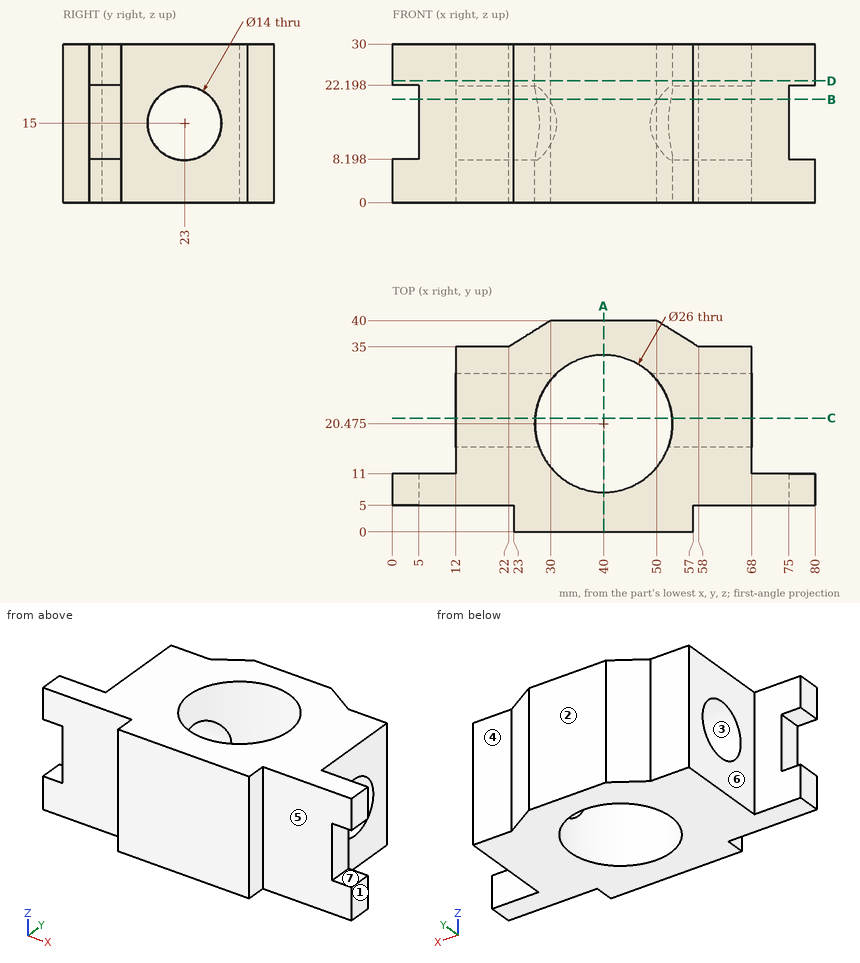
Check sheet for the drawn part. Datum: minimum x, y, z corner. Units: mm. A direction names the side the tool comes from. Coordinates: 2 decimals unless noted, no trailing zeros. Loops run counter-clockwise (first coordinate to the right, second up) from the corner with the lowest first, then second, coordinate; pieces in that order, holes last. Notation, with made-up numbers: (-26.5, 81.25) -> (-20.5, 81.25) arc R16 cw to (-20.5, 103.25) -> close; hole circle Ø7 at (44, -38.75). An arc over 180 degrees is marked (long way). Write each question's results on one line, items separated by ' | '.
Item 1: Mould release check, pull along Y, two halves, no side actions. Record for the marked faces 1, 2 and 3: +Y half, -Y half, draft (parallel to the pull), parting line (faces both ways), or undercut.
Found:
face 1: draft | face 2: +Y half | face 3: undercut
Item 2: Tool access check on the marked faces 4, 5, 6 and 7. Record the directions out of +Z, -Z, +X, -X, +Y, -Y that give a thin tool (end or side, any length) a straight path to the whole face; none if there is none.
Found:
face 4: +Z, -Z, +X, +Y | face 5: +Z, -Z, +X, -Y | face 6: +Z, -Z, -X, +Y | face 7: +X, +Y, -Y
Item 3: Section check C-C, the plane y = 21.5. Enter the section's corners in (x, z).
Found:
outline: (12, 0) -> (27.04, 0) -> (27.04, 8.16) -> (12, 8.16) -> close; (12, 21.84) -> (27.04, 21.84) -> (27.04, 30) -> (12, 30) -> close; (52.96, 0) -> (68, 0) -> (68, 8.16) -> (52.96, 8.16) -> close; (52.96, 21.84) -> (68, 21.84) -> (68, 30) -> (52.96, 30) -> close
Item 4: Material ranges on L1, parallel to Y at x = 40, z = 16 (1 decimal); L2, parallel to Z at x = 21, y = 23; L3, parallel to Y at x = 19.5, z = 25, recorded low to high.
Found:
L1: y = 0 to 7.5, 33.5 to 40 | L2: z = 0 to 8, 22 to 30 | L3: y = 5 to 35
Item 5: Section check A-A, the plane x = 40. Enter the section's corners in (y, z) (1 decimal).
Found:
outline: (0, 0) -> (7.5, 0) -> (7.5, 30) -> (0, 30) -> close; (33.5, 0) -> (40, 0) -> (40, 30) -> (33.5, 30) -> close
Item 6: Section check D-D, the plane z = 23. Enter the section's corners in (x, y) (1 decimal), plus the area to 3 significant figures.
Found:
outline: (0, 5) -> (23, 5) -> (23, 0) -> (57, 0) -> (57, 5) -> (80, 5) -> (80, 11) -> (68, 11) -> (68, 35) -> (58, 35) -> (50, 40) -> (30, 40) -> (22, 35) -> (12, 35) -> (12, 11) -> (0, 11) -> close; hole circle Ø26 at (40, 20.5) | area: 1,600 mm2
Item 7: Gauge pin test, flat ends, axial feed: pin 1 (10 mm diameter, centred on y = 25, z = 9.5, fed in from -X); pin 2 (5 mm diameter, centred on y = 7, z = 15, fed in from +X); pin 3 (11.5 mm diameter, centred on x = 7, z = 19, fed in from -Y). Record the tip position at first contact, or that the pin passes through.
Found:
pin 1: stops at x = 12 | pin 2: stops at x = 75 | pin 3: stops at y = 5
Item 8: Section check B-B, the plane z = 19.5. Enter the section's corners in (x, y) (1 decimal), plus the area to 3 significant figures.
Found:
outline: (5, 5) -> (23, 5) -> (23, 0) -> (57, 0) -> (57, 5) -> (75, 5) -> (75, 11) -> (68, 11) -> (68, 17.6) -> (52.7, 17.6) arc R13 cw to (27.3, 17.6) -> (12, 17.6) -> (12, 11) -> (5, 11) -> close; (12, 28.4) -> (29.7, 28.4) arc R13 cw to (50.3, 28.4) -> (68, 28.4) -> (68, 35) -> (58, 35) -> (50, 40) -> (30, 40) -> (22, 35) -> (12, 35) -> close | area: 1,210 mm2
